Autodesk Inventor part; units mm, degrees
ref_plane "YZ Plane" through (0, 0, 0) normal (1, 0, 0) x (0, 1, 0)
ref_plane "XZ Plane" through (0, 0, 0) normal (0, 1, 0) x (-1, 0, 0)
ref_plane "XY Plane" through (0, 0, 0) normal (0, 0, 1) x (1, 0, 0)
sketch "Sketch1" plane through (0, 0, 0) normal (0, 0, 1) x (1, 0, 0)
  line L0 (0, 0) -> (100, 0)
  line L1 (100, 0) -> (100, -45)
  line L2 (100, -45) -> (0, -45)
  line L3 (0, -45) -> (0, 0)
  dimension "d0" = 100
  dimension "d1" = 45
extrude "Extrusion1" add sketch "Sketch1" along normal blind 5
sketch "Sketch2" plane through (0, 0, 0) normal (0, 0, -1) x (-1, 0, 0)
  point P0 (0, 0)
  point P1 (-15, -22.5)
  point P2 (-85, -22.5)
  dimension "d4" = 70
  dimension "d5" = 15
  dimension "d6" = 22.5
hole "Hole1" at (15, -22.5, 0) at (85, -22.5, 0) direction (0, 0, 1) diameter 4 depth 5 tip angle 118 counterbore diameter 8 counterbore depth 2.5
properties part number "as3"
Input: part model. Units: mm. Frame: model coordinates. A direction names the side the tool comes from. Coordinates: 2 decimals unless noted, no trailing zeros. Order: outer loops, then holes, each group sorted by start corner. A loop starts at its lowest first (then second) coordinate and runs counter-clockwise, first axis right, second up. Notation, with made-up numbers: M -24,33 L -1,33 A30 cw -1,66 Z; hole C 52.5,23.25 d7. An arc over 180 degrees is marked long. Write item = value, one per line. Start each with the question number.
(1) Line query: line 1 along X through (y, z) = (-22.5, 3.55); line 2 along X through (y, z) = (-22.5, 1.5); line 3 along Y through (x, z) = (85, 0.9). Output: solid intervals per line, ascending. Write a range as [from, to].
(2) First-contact query: P1, Ø6.5, axis at x = 15.5, y = -22.5, coming from the -Z side. Flat tip, straight axial feed; report the tip coordinate or a pass-through.
(3) Section A-A on y = -22.5. Output: boundary loops of the cut face in (x, z).
(4) Pull-direction query (Y, two-part tool) for faces 1 (the flat face through (0, -23, 2)), 2 (the flat face through (49, 0, 2)), 3 (the cylindrical face through (13.017, -22.76, 3.768)); classes: released by +Y, released by -Y, zero draft, split by the parting line, or undercut.
(5) Section B-B on x = 15. Output: boundary loops of the cut face in (y, z), and give its area (3 significant figures).
(6) Reachability of faces 4 (the cylindrical face through (83.017, -22.76, 3.768)), 5 (the cylindrical face through (88.905, -23.367, 1.268)) from +Z, -Z, +X, -X, +Y, -Y: full face, straight path, thin tool, end or side. Return the list, or none.
Result set:
q1.line_1 = [0, 13], [17, 83], [87, 100]
q1.line_2 = [0, 11], [19, 81], [89, 100]
q1.line_3 = [-45, -26.5], [-18.5, 0]
q2.P1 = 2.5
q3.outline = M 0,0 L 11,0 L 11,2.5 L 13,2.5 L 13,5 L 0,5 Z; M 17,2.5 L 19,2.5 L 19,0 L 81,0 L 81,2.5 L 83,2.5 L 83,5 L 17,5 Z; M 87,2.5 L 89,2.5 L 89,0 L 100,0 L 100,5 L 87,5 Z
q4.face_1 = zero draft
q4.face_2 = released by +Y
q4.face_3 = undercut
q5.outline = M -45,0 L -26.5,0 L -26.5,2.5 L -24.5,2.5 L -24.5,5 L -45,5 Z; M -20.5,2.5 L -18.5,2.5 L -18.5,0 L 0,0 L 0,5 L -20.5,5 Z
q5.area = 195 mm²
q6.face_4 = +Z, -Z
q6.face_5 = -Z
